Here's how the part is built. I have some questions about the finished solid (model axes, mm). Face numbers are marked on the shaded views. Round coordinates to 2 decimals unless told otherwise and drop trailing zeros. Write each loop counter-clockwise with the first axis right and the second up, starting at its lowest first coordinate (ties: lowest second). Pieces come first, ordered by that corner, then holes. Notation, with made-up numbers: (45, -24) -> (95, -24) arc R18 cw to (95, -13) -> close; hole circle Ø3 at (-18, 62.5). An arc over 180 degrees is marked (long way). Put each result on its own line as item: value. Start each with the question number.
1) We'd pull the mould along Z, two halves only. Please class the marked faces 1, 2 and 3: released by +Z, released by -Z, zero draft, split by the parting line, or undercut.
2) I want a section at A-A, the plane y = -23. List the corners of the cut face in (x, z) for me, then the cut area to 3 significant figures.
3) Will these pins go through, and if not, where does the flat tip stop? P1, Ø4, axis at x = -72.5, z = -103.5, coming from the +Y side; P2, Ø4, axis at x = 68.5, z = -149, coming from the -Y side; P3, Ø8, axis at x = 81, z = -192, coming from the +Y side.
4) If I drill on line 1 along Z through (x, y) = (-2, -22); line 2 along X through (y, z) = (-24, -158); line 3 along Z through (x, y) = (-101.5, -36), over which ranges is the centre line in solid material (lowest first)? Write a range as [from, to].
5) I want a section at B-B, the plane y = 5. List the corners of the cut face in (x, z) for me, then the cut area to 3 significant figures.
Autodesk Inventor part; units mm, degrees
ref_plane "YZ Plane" through (0, 0, 0) normal (1, 0, 0) x (0, 1, 0)
ref_plane "XZ Plane" through (0, 0, 0) normal (0, 1, 0) x (-1, 0, 0)
ref_plane "XY Plane" through (0, 0, 0) normal (0, 0, 1) x (1, 0, 0)
sketch "Sketch1" plane through (0, 0, 0) normal (1, 0, 0) x (0, 1, 0)
  line L0 (16.3991, -98.278) -> (51.3241, -72.878) construction
  line L1 (51.3241, -72.878) -> (51.3241, -74.402) construction
  line L2 (51.3241, -74.402) -> (16.3991, -99.802) construction
  line L3 (0, -113.538) -> (16.3991, -113.538)
  line L4 (0, 0.762) -> (0, -0.762)
  line L5 (0, 0.762) -> (16.3991, -98.278)
  line L6 (0, -0.762) -> (16.3991, -99.802)
  line L7 (16.3991, -99.802) -> (16.3991, -98.278)
  line L8 (16.3991, -98.278) -> (33.1367, -86.1052) construction
  line L9 (33.1367, -86.1052) -> (19.6348, -72.4523) construction
  spline S0 degree 2 poles (16.3991, -98.278) (33.1367, -86.1052) (19.6348, -72.4523) knots 1 1 1 2 2 2
  line L10 (19.6348, -72.4523) -> (20.7184, -71.3806)
  line L11 (16.3991, -99.802) -> (33.8616, -87.102) construction
  line L12 (33.8616, -87.102) -> (21.7781, -72.4523) construction
  spline S1 degree 2 poles (16.3991, -99.802) (33.8616, -87.102) (21.7781, -72.4523) knots 1 1 1 2 2 2
  line L13 (21.7781, -72.4523) -> (20.7184, -71.3806)
  line L14 (0, 0.762) -> (-44.45, 0.762)
  line L15 (-44.45, 0.762) -> (-44.45, -0.762)
  line L16 (-44.45, -0.762) -> (0, -0.762)
  line L17 (0, -0.762) -> (0, 0.762)
  point P0 (0, 0)
  dimension "d5" = 1.524
  dimension "d8" = 34.925
  dimension "d26" = 1.524
  dimension "d27" = 1.524
  dimension "d28" = 1.524
  dimension "d30" = 44.45
  dimension "d31" = 1.524
  dimension "d32" = 114.3
revolve "Revolution2" add sketch "Sketch1" angle 360 about axis through (0, 0, -113.538) along (0, 1, 0)
properties part number "rubber_sleeve" material "Rubber"
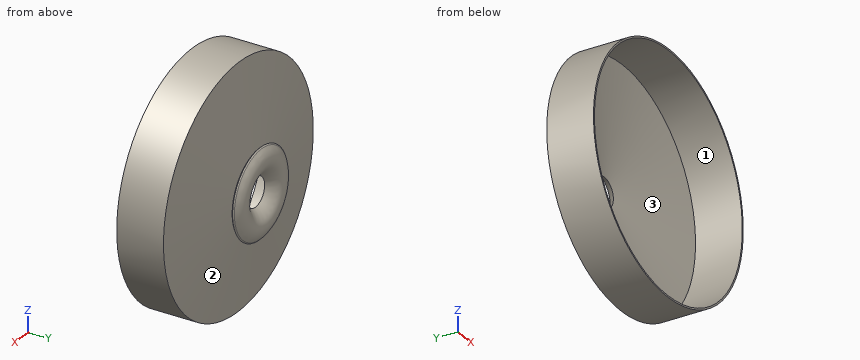
Findings:
1. face 1: undercut
1. face 2: split by the parting line
1. face 3: undercut
2. outline: circle Ø228.6 at (0, -113.54); hole circle Ø225.55 at (0, -113.54)
2. area: 1,090 mm2
3. P1: stops at y = 7.14
3. P2: stops at y = 5.57
3. P3: stops at y = 0.92
4. line 1: z = [-227.82, -226.3], [-0.78, 0.74]
4. line 2: x = [-105.3, -103.64], [103.64, 105.3]
4. line 3: z = [-166.1, -162.69], [-64.38, -60.98]
5. outline: circle Ø168.21 at (0, -113.54); hole circle Ø165.16 at (0, -113.54)
5. area: 798 mm2
